Read the model definition and answer for the solid it produces. Units are mm, in the model's axes. A direction names the side the tool comes from. Coordinates: 2 decimals unless noted, no trailing zeros. Loops run counter-clockwise (first coordinate to the right, second up) from the corner with the lowest first, then second, coordinate; pieces in that order, holes last.
from build123d import *

# Parameters (mm, degrees)
SKETCH1_W           = 29.337
SKETCH1_H           = 15.367
BOSS_EXTRUDE1_DEPTH = 19.2024
SKETCH2_R           = 5.9055
BOSS_EXTRUDE2_DEPTH = 9.144
SKETCH3_W           = 6.35
SKETCH3_H           = 6.35
BOSS_EXTRUDE3_DEPTH = 7.62
SKETCH4_R           = 2.8321


with BuildPart() as part:
    # Sketch1 → Boss-Extrude1 (new body)
    with BuildSketch(Plane(origin=(0, 0, 0), x_dir=(1, 0, 0), z_dir=(0, 1, 0))):
        Rectangle(SKETCH1_W, SKETCH1_H)
    extrude(amount=BOSS_EXTRUDE1_DEPTH)

    # Sketch2 → Boss-Extrude2 (add)
    with BuildSketch(Plane(origin=(0, 19.2024, 0), x_dir=(1, 0, 0), z_dir=(0, 1, 0))):
        Circle(SKETCH2_R)
    extrude(amount=BOSS_EXTRUDE2_DEPTH)

    # Sketch3 → Boss-Extrude3 (add)
    with BuildSketch(Plane.XZ):
        with Locations((-11.4935, 0)):
            Rectangle(SKETCH3_W, SKETCH3_H)
        with Locations((11.4935, 0)):
            Rectangle(SKETCH3_W, SKETCH3_H)
    extrude(amount=BOSS_EXTRUDE3_DEPTH)

    # Sweep1: sweep along a path in Sketch5
    with BuildLine(Plane.XY) as sweep1_path:
        Line((0, 28.3464), (-3.175, 45.840621189))
    # Sketch4 → Sweep1 (sweep)
    with BuildSketch(Plane(origin=(0, 28.3464, 0), x_dir=(1, 0, 0), z_dir=(0, 1, 0))):
        Circle(SKETCH4_R)
    sweep(path=sweep1_path.line)


solid = part.part
Q1. Which of the six approach directions +Z, -Z, +X, -X, +Y, -Y give full straight-line access (tool end or side, diameter ignored) to faces 5 (the face through (-8.318, -4, 0)), 6 (the face through (0, 9, 7.684)), 7 (the face through (11, -4, 3.175)), 8 (the face through (3, 28.346, -1)), 9 (the face through (-12, -4, -3.175))?
Findings below:
face 5: +Z, -Z, -Y
face 6: +Z, +X, -X, +Y, -Y
face 7: +Z, +X, -X, -Y
face 8: none
face 9: -Z, +X, -X, -Y
Q2. A cutting plane is placed at B-B (y = 21). Give the vertices of the cut face in (x, z), then the cut area to 3 significant figures.
Findings below:
outline: circle Ø11.81 at (0, 0)
area: 110 mm2
Q3. A cutting plane is placed at A-A (z = 5.25). Give the vertices of the cut face in (x, y), then the cut area to 3 significant figures.
Findings below:
outline: (-14.67, 0) - (14.67, 0) - (14.67, 19.2) - (2.7, 19.2) - (2.7, 28.35) - (-2.7, 28.35) - (-2.7, 19.2) - (-14.67, 19.2) - close
area: 613 mm2
Q4. A cutting plane is placed at C-C (x = 4.5). Give the vertices of the cut face in (y, z).
Findings below:
outline: (0, -7.68) - (19.2, -7.68) - (19.2, -3.82) - (28.35, -3.82) - (28.35, 3.82) - (19.2, 3.82) - (19.2, 7.68) - (0, 7.68) - close
Q5. A cutting plane is placed at D-D (x = -7.75). Give the vertices of the cut face in (y, z).
Findings below:
outline: (0, -7.68) - (19.2, -7.68) - (19.2, 7.68) - (0, 7.68) - close
Q6. Determine the mould class of faces 1 (the face through (11, -7.62, 0)), 2 (the face through (-4.69, 23.71, 3.59)), 3 (the face through (14.668, 9, 0)), 4 (the face through (8.318, -4, 0)) for opening direction X: +X half, -X half, draft (parallel to the pull), parting line (faces both ways), or undercut.
Findings below:
face 1: draft
face 2: parting line
face 3: +X half
face 4: undercut
Q7. Straight lines are drawn through the part: probe 1 along Y at (x, z) = (-2.75, 0); probe 2 along Y at (x, z) = (-6.5, 4.5); probe 3 along Z at (x, y) = (-4, 19.5). For each, find the intervals that lie inside material, in ascending order.
Findings below:
probe 1: y = 0 to 45.84
probe 2: y = 0 to 19.2
probe 3: z = -4.34 to 4.34
Q8. Flat-ended cylindrical pins translate along their axes: pin 1 Ø5 at (x, z) = (-6, 5.5) entering from +Y; pin 2 Ø3 at (x, y) = (-11.5, -5) entering from -Z (3 decimals); pin 3 Ø6 at (y, z) = (33, -5) entering from +X. Find the tip coordinate at first contact, or state that the pin passes through.
Findings below:
pin 1: stops at y = 28.35
pin 2: stops at z = -3.175
pin 3: stops at x = 1.21
